Input: part model. Units: mm. Frame: model coordinates. A direction names the side the tool comes from. Coordinates: 2 decimals unless noted, no trailing zeros. Order: outer loops, then holes, each group sorted by start corner. A loop starts at its lowest first (then second) coordinate and runs counter-clockwise, first axis right, second up. Notation, with made-up numbers: (-4, 15.25) - (40, 15.25) arc R13 ccw to (40, 26.25) - close; hole circle Ø5 at (-32.75, 66.5). An arc over 180 degrees is marked (long way). Answer as CSV lines item,"result". Start each with the question number.
Item 1: Section C-C (y = -31). Output: boundary loops of the cut face in (x, z), and give its area (3 significant figures).
Item 2: Section B-B (z = 0). Output: boundary loops of the cut face in (x, y), and give its area (3 significant figures).
Item 3: First-contact query: pin 1 (1.5 mm diameter, centred on y = -23, z = -1.5, fed in from -X); pin 2 (1 mm diameter, centred on x = 1.5, y = -13, fed in from +Z). Flat tips, straight axial feed; report the tip coordinate or a pass-through.
Item 4: Section A-A (x = 0). Output: boundary loops of the cut face in (y, z).
Item 5: Access query for faces 1 (the flat face through (0, 0, 0)), 2 (the cylindrical face through (0, -4, -2)), 3 (the cylindrical face through (0, -69, -2)). Directions: +Z, -Z, +X, -X, +Y, -Y. A direction counts if a zero-diameter tool reaches every point of the face in a straight line with its end or side. Return the directions, or none.
Item 6: Material intervals for line 1 along Z through (x, y) = (-1, -46.5); line 2 along Y through (x, z) = (1.3, -1.55); line 3 along X through (y, z) = (-38.5, -1.6), sorted ascending.
from build123d import *

# Parameters (mm, degrees)
F0_R     = 2
F1_DEPTH = 7.5
F2_R     = 2.25
F2_R_2   = 2
F3_DEPTH = 58
F4_R     = 2
F5_DEPTH = 7.5


with BuildPart() as f1:
    # F0 (on Front) → F1 (new body)
    with BuildSketch(Plane.XZ):
        Circle(F0_R)
    extrude(amount=F1_DEPTH)

    # F2 (on face) → F3 (join)
    with BuildSketch(Plane.XZ.offset(7.5)):
        Circle(F2_R)
        Circle(F2_R_2, mode=Mode.SUBTRACT)
        Circle(F2_R_2)
    extrude(amount=F3_DEPTH)

    # F4 (on face) → F5 (join)
    with BuildSketch(Plane.XZ.offset(65.5)):
        Circle(F4_R)
    extrude(amount=F5_DEPTH)


solid = f1.part
Determined:
1,outline,"circle Ø4.5 at (0, 0)"
1,area,"15.9 mm^2"
2,outline,"(-2.25, -65.5) - (-2, -65.5) - (-2, -73) - (2, -73) - (2, -65.5) - (2.25, -65.5) - (2.25, -7.5) - (2, -7.5) - (2, 0) - (-2, 0) - (-2, -7.5) - (-2.25, -7.5) - close"
2,area,"321 mm^2"
3,pin 1,"stops at x = -2.12"
3,pin 2,"stops at z = 2.02"
4,outline,"(-73, -2) - (-65.5, -2) - (-65.5, -2.25) - (-7.5, -2.25) - (-7.5, -2) - (0, -2) - (0, 2) - (-7.5, 2) - (-7.5, 2.25) - (-65.5, 2.25) - (-65.5, 2) - (-73, 2) - close"
5,face 1,"+Z, -Z, +X, -X, +Y"
5,face 2,"+Y"
5,face 3,"-Y"
6,line 1,"z = -2.02 to 2.02"
6,line 2,"y = -65.5 to -7.5"
6,line 3,"x = -1.58 to 1.58"
